```python
from build123d import *

# Parameters (mm, degrees)
F0_W     = 40
F0_H     = 40
F0_R     = 12.5
F1_DEPTH = 40
F2_R     = 12.5
F3_DEPTH = 40.001


with BuildPart() as f1:
    # F0 (on Top) → F1 (new body)
    with BuildSketch(Plane.XY):
        Rectangle(F0_W, F0_H)
        Circle(F0_R, mode=Mode.SUBTRACT)
    extrude(amount=F1_DEPTH)

    # F2 (on face) → F3 (cut, through all)
    with BuildSketch(Plane.XZ.offset(20)):
        with Locations((0, 20)):
            Circle(F2_R)
    extrude(amount=-F3_DEPTH, mode=Mode.SUBTRACT)


solid = f1.part
```
Source: CAD feature listing. Evaluate the final solid. Frame: model axes, mm. Round coordinates to 2 decimals unless told otherwise and drop trailing zeros. Write each loop counter-clockwise with the first axis right and the second up, starting at its lowest first coordinate (ties: lowest second). Pieces come first, ordered by that corner, then holes. Notation, with made-up numbers: M -2.5,-5.75 L 54.5,-5.75 A20 ccw 54.5,7.25 Z; hole C -6,1.5 d2. An arc over 180 degrees is marked long. Answer as a JSON object with one key per item and string values. Group by question number.
(1) Section query C-C on z = 4.5. Output: boundary loops of the cut face in (x, y).
(2) Ray query, line 1 (X direction, y = 10, z = 20); line 2 (X direction, y = -11.5, z = 11). Return the intervals inside material, ascending. Write a range as [from, to].
(3) Section query D-D on x = -7. Output: boundary loops of the cut face in (y, z).
(4) Section query B-B on y = 3.5. Output: boundary loops of the cut face in (x, z).
(5) First-contact query: pin 1 (10 mm diameter, centred on x = 11, y = -3, fed in from +Z). Flat tip, straight axial feed; report the tip coordinate or a pass-through.
(6) Mould query, pull axis Y, two halves, no side actions, for faces 1 (the flat face through (-9, 20, 11)), 2 (the cylindrical face through (-9.92, -7.606, 7.638)), 3 (the flat face through (-9, 9, 40)). Classes: +Y half, -Y half, draft (parallel to the pull), parting line (faces both ways), or undercut.
(7) Section query A-A on x = 0. Output: boundary loops of the cut face in (y, z).
Computed values:
{
 "1": {"outline": "M -20,-20 L 20,-20 L 20,20 L -20,20 Z; hole C 0,0 d25"},
 "2": {"line 1": "[-20, -12.5], [12.5, 20]", "line 2": "[-20, -8.67], [8.67, 20]"},
 "3": {"outline": "M -20,0 L -10.36,0 L -10.36,9.64 L -20,9.64 Z; M -20,30.36 L -10.36,30.36 L -10.36,40 L -20,40 Z; M 10.36,0 L 20,0 L 20,9.64 L 10.36,9.64 Z; M 10.36,30.36 L 20,30.36 L 20,40 L 10.36,40 Z"},
 "4": {"outline": "M -20,0 L -12,0 L -12,16.5 A12.5 cw -12,23.5 L -12,40 L -20,40 Z; M 12,0 L 20,0 L 20,40 L 12,40 L 12,23.5 A12.5 cw 12,16.5 Z"},
 "5": {"pin 1": "z = 40"},
 "6": {"face 1": "+Y half", "face 2": "undercut", "face 3": "draft"},
 "7": {"outline": "M -20,0 L -12.5,0 L -12.5,7.5 L -20,7.5 Z; M -20,32.5 L -12.5,32.5 L -12.5,40 L -20,40 Z; M 12.5,0 L 20,0 L 20,7.5 L 12.5,7.5 Z; M 12.5,32.5 L 20,32.5 L 20,40 L 12.5,40 Z"}
}
